Source: CAD feature listing. Evaluate the final solid. Frame: model axes, mm. Give positions to 0.01 mm unless a question says otherwise; leave off trailing zeros. Order: outer loops, then holes, each group sorted by start corner. A loop starts at its lowest first (then second) coordinate and runs counter-clockwise, first axis right, second up. Notation, with made-up numbers: M 39,74.25 L 98,74.25 A18 ccw 98,93.25 Z; hole C 53,45 d4. An arc over 180 degrees is marked long. Answer as a JSON object with one key per item and string values. Group by question number.
1. Material intervals for L1, parallel to Y at x = -0.15, z = -0.05; L2, parallel to X at y = 15, z = 1.35; L3, parallel to X at y = 27.5, z = -2.35, sorted ascending. Write a range as [from, to].
2. Section query C-C (y = 29.5). Output: boundary loops of the cut face in (x, z).
3. Pin query (flat end, axial travel): P1, Ø1, axis at x = 2, y = 7.5, coming from the -Z side; P2, Ø1.5, axis at x = 0, z = 2.5, coming from the -Y side; P3, Ø2, axis at x = 2, z = 1.5, coming from the -Y side. Return the tip coordinate at first contact, or that it passes through.
4. Section query A-A (x = 0). Output: boundary loops of the cut face in (y, z), plus the area to 3 significant figures.
5. Section query B-B (z = -0.55). Output: boundary loops of the cut face in (x, y).
from build123d import *

# Parameters (mm, degrees)
SKETCH1_R           = 3
BOSS_EXTRUDE1_DEPTH = 52
DOME1_FACE_RADIUS   = 3
DOME1_HEIGHT        = 2
DOME2_FACE_RADIUS   = 3
DOME2_HEIGHT        = 2


with BuildPart() as part:
    # Sketch1 → Boss-Extrude1 (new body)
    with BuildSketch(Plane(origin=(0, 0, 0), x_dir=(1, 0, 0), z_dir=(0, 1, 0))):
        Circle(SKETCH1_R)
    extrude(amount=BOSS_EXTRUDE1_DEPTH)

    # Dome1: a dome of height H over a round flat face of radius A is a cap of a sphere of radius (A * A + H * H) / (2 * H)
    dome1_r = (DOME1_FACE_RADIUS * DOME1_FACE_RADIUS + DOME1_HEIGHT * DOME1_HEIGHT) / (2 * DOME1_HEIGHT)
    dome1_base = Plane((0, 52, 0), z_dir=(0, 1, 0))
    with Locations(dome1_base.offset(DOME1_HEIGHT - dome1_r)):
        dome1_ball = Sphere(dome1_r, mode=Mode.PRIVATE)
    add(split(dome1_ball, bisect_by=dome1_base, keep=Keep.TOP, mode=Mode.PRIVATE))

    # Dome2: a dome of height H over a round flat face of radius A is a cap of a sphere of radius (A * A + H * H) / (2 * H)
    dome2_r = (DOME2_FACE_RADIUS * DOME2_FACE_RADIUS + DOME2_HEIGHT * DOME2_HEIGHT) / (2 * DOME2_HEIGHT)
    dome2_base = Plane((0, 0, 0), z_dir=(0, -1, 0))
    with Locations(dome2_base.offset(DOME2_HEIGHT - dome2_r)):
        dome2_ball = Sphere(dome2_r, mode=Mode.PRIVATE)
    add(split(dome2_ball, bisect_by=dome2_base, keep=Keep.TOP, mode=Mode.PRIVATE))


solid = part.part
Answer sheet:
{
 "1": {"L1": "[-2, 54]", "L2": "[-2.68, 2.68]", "L3": "[-1.86, 1.86]"},
 "2": {"outline": "C 0,0 d6"},
 "3": {"P1": "z = -2.6", "P2": "y = -1.49", "P3": "y = -1.63"},
 "4": {"outline": "M 0,-3 L 52,-3 A3.25 ccw 52,3 L 0,3 A3.25 ccw Z", "area": "329 mm^2"},
 "5": {"outline": "M -2.95,0 A3.2 ccw 2.95,0 L 2.95,52 A3.2 ccw -2.95,52 Z"}
}
